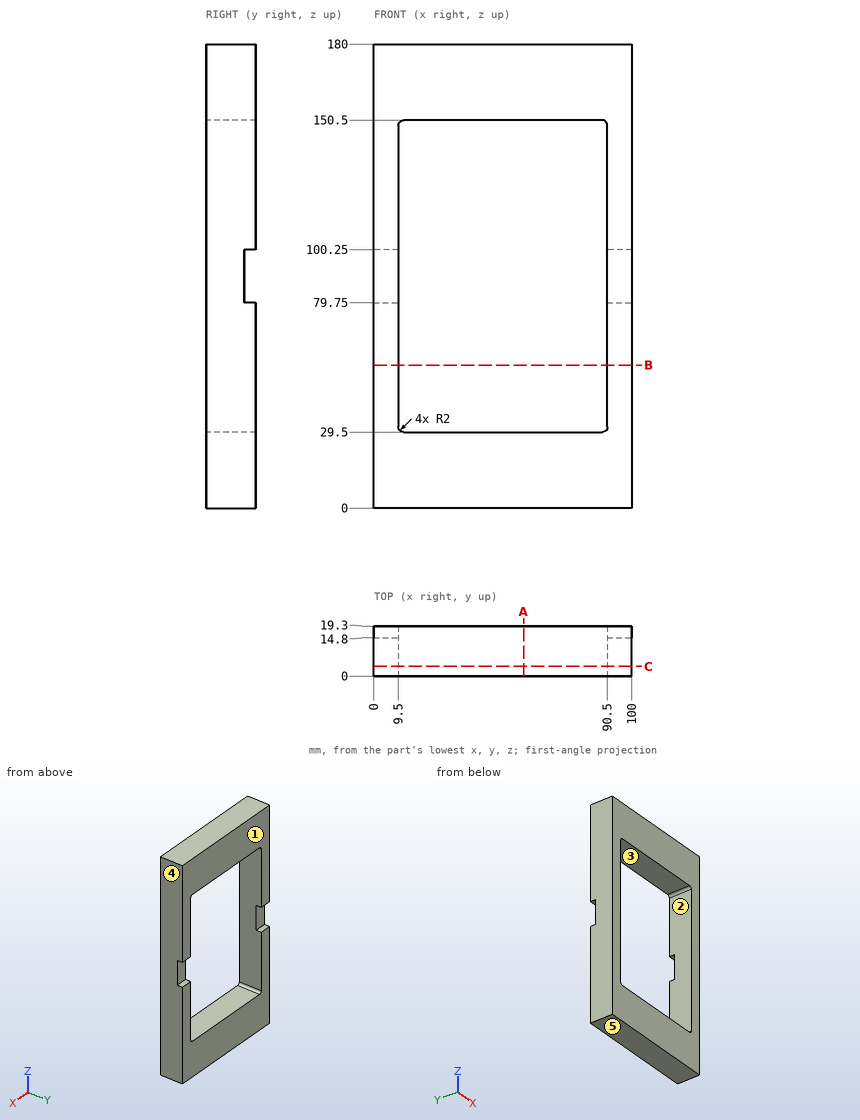
Part print with two shaded views. Sizes in mm from the minimum x, y, z corner. A direction names the side the tool comes from. Round coordinates to 2 decimals unless told otherwise and drop trailing zeros. Write each loop counter-clockwise with the first axis right and the second up, starting at its lowest first coordinate (ties: lowest second). Pieces come first, ordered by that corner, then holes. Notation, with made-up numbers: M 21,9 L 51,9 A23 cw 51,32 Z; hole C 44.5,48.25 d3. An arc over 180 degrees is marked long. Answer as CSV lines item,"result". Start each with the question number.
1) Band-saw the part on B-B (z = 55.5). List the corners of the cut face in (x, y).
2) Which spindle directions (+Z, -Z, +X, -X, +Y, -Y) get a long thin tool onto all of the face, cutting with end or side? Do the marked faces 1 and 2. Say none if no direction does.
3) Band-saw the part on A-A (x = 58). List the corners of the cut face in (y, z), then the cut area to 3 significant figures.
4) Drill centre lines: L1, parallel to X at y = 17.25, z = 57.5; L2, parallel to Z at x = 69.5, y = 11.75; L3, parallel to Z at x = 7, y = 16.5. Where is each one in solid material? Low to high.
5) Drop flat-ended pins along their axis: pin 1 (1.3 mm diameter, centred on x = 4.5, y = 17, fed in from -Z); pin 2 (10.5 mm diameter, centred on x = 3, z = 90, fed in from +Y). Give the stop position or say it passes through.
6) Band-saw the part on C-C (y = 3.75). List the corners of the cut face in (x, z), then the cut area to 3 significant figures.
7) Mould opens along X. For the marked faces 3, 4 and 5 say: +X half, -X half, draft (parallel to the pull), parting line (faces both ways), or undercut.
Worked out:
1,outline,"M 0,0 L 9.5,0 L 9.5,19.3 L 0,19.3 Z; M 90.5,0 L 100,0 L 100,19.3 L 90.5,19.3 Z"
2,face 1,"+Z, -Z, +X, -X, +Y"
2,face 2,"+Y, -Y"
3,outline,"M 0,0 L 19.3,0 L 19.3,29.5 L 0,29.5 Z; M 0,150.5 L 19.3,150.5 L 19.3,180 L 0,180 Z"
3,area,"1,140 mm²"
4,L1,"0 to 9.5, 90.5 to 100"
4,L2,"0 to 29.5, 150.5 to 180"
4,L3,"0 to 79.75, 100.25 to 180"
5,pin 1,"z = 0"
5,pin 2,"y = 14.8"
6,outline,"M 0,0 L 100,0 L 100,180 L 0,180 Z; hole M 9.5,31.5 A2 ccw 11.5,29.5 L 88.5,29.5 A2 ccw 90.5,31.5 L 90.5,148.5 A2 ccw 88.5,150.5 L 11.5,150.5 A2 ccw 9.5,148.5 Z"
6,area,"8,200 mm²"
7,face 3,"undercut"
7,face 4,"+X half"
7,face 5,"draft"
